```python
from build123d import *

# Parameters (mm, degrees)
SKETCH1_W           = 406.4
SKETCH1_H           = 184.15
BOSS_EXTRUDE1_DEPTH = 12.7
SKETCH2_R           = 12.5
CUT_EXTRUDE1_DEPTH  = 5
FILLET1_R           = 5


with BuildPart() as part:
    # Sketch1 → Boss-Extrude1 (new body)
    with BuildSketch(Plane(origin=(0, 0, 0), x_dir=(1, 0, 0), z_dir=(0, 1, 0))):
        with Locations((203.2, 92.075)):
            Rectangle(SKETCH1_W, SKETCH1_H)
    extrude(amount=BOSS_EXTRUDE1_DEPTH)

    # Sketch2 → Cut-Extrude1 (cut)
    with BuildSketch(Plane(origin=(0, 12.7, 0), x_dir=(1, 0, 0), z_dir=(0, 1, 0))):
        with Locations(Location((29.195557492, 20, 0), (0, 0, 270))):
            Circle(SKETCH2_R)
        with Locations(Location((377.204442508, 20, 0), (0, 0, 270))):
            Circle(SKETCH2_R)
        with Locations(Location((377.204442508, 164.15, 0), (0, 0, 270))):
            Circle(SKETCH2_R)
        with Locations(Location((29.195557492, 164.15, 0), (0, 0, 270))):
            Circle(SKETCH2_R)
    extrude(amount=-CUT_EXTRUDE1_DEPTH, mode=Mode.SUBTRACT)

    # Fillet1
    fillet1_edges = [part.edges().sort_by_distance(p)[0] for p in [
        (29.195557492, 7.7, -176.65),
        (377.204442508, 7.7, -176.65),
        (377.204442508, 7.7, -32.5),
        (29.195557492, 7.7, -32.5),
    ]]
    fillet(fillet1_edges, radius=FILLET1_R - 0.0001)  # a hair under: the kernel refuses the full size


solid = part.part
```
The model under review builds one solid part; all positions refer to its coordinate system, in mm. A direction names the side the tool comes from. Round coordinates to 2 decimals unless told otherwise and drop trailing zeros. Use CSV: the item, a comma, the result in double quotes. Start each with the question number.
(1) The part is to be moulded in two halves that separate along Z. For faces 3 (the face through (200, 6, 0)), 4 (the face through (377, 7.7, -164)), 5 (the face through (406.4, 6, -91)), say which applies: +Z half, -Z half, draft (parallel to the pull), parting line (faces both ways), or undercut.
(2) Tool access review of faces 1 (the face through (200, 0, -93)), 2 (the face through (377, 7.7, -20)): name each direction out of +Z, -Z, +X, -X, +Y, -Y from which nothing blocks a thin tool from reaching the whole face with its end or side.
(3) Clearance check with flat-ended pins moving along their axes: P1, Ø12, axis at x = 31.5, z = -165.5, coming from the +Y side; P2, Ø12, axis at x = 378, z = -16.5, coming from the +Y side; P3, Ø12, axis at x = 32, z = -23, coming from the +Y side. State where each tip first meets the part, or that it passes through.
(4) For line 1 along X through (y, z) = (11.5, -175.5); line 2 along Y through (x, z) = (373, -169), list the stretches that pass through material, from the lowest coordinate up.
Findings:
1,face 3,"+Z half"
1,face 4,"undercut"
1,face 5,"draft"
2,face 1,"+Z, -Z, +X, -X, -Y"
2,face 2,"+Y"
3,P1,"y = 7.84"
3,P2,"y = 8.16"
3,P3,"y = 8.43"
4,line 1,"0 to 24.32, 34.07 to 372.33, 382.08 to 406.4"
4,line 2,"0 to 7.7"
